Autodesk Inventor part; units mm, degrees
ref_plane "YZ Plane" through (0, 0, 0) normal (1, 0, 0) x (0, 1, 0)
ref_plane "XZ Plane" through (0, 0, 0) normal (0, 1, 0) x (-1, 0, 0)
ref_plane "XY Plane" through (0, 0, 0) normal (0, 0, 1) x (1, 0, 0)
sketch "Sketch1" plane through (0, 0, 0) normal (0, 1, 0) x (-1, 0, 0)
  circle A0 centre (0, 0) radius 1.1
  dimension "d0" = 2.2
extrude "Extrusion1" add sketch "Sketch1" along normal blind 16
sketch "Sketch2" plane through (0, 16, 0) normal (0, 1, 0) x (1, 0, 0)
  circle A0 centre (0, 0) radius 1.85
  dimension "d3" = 3.7
extrude "Extrusion2" add sketch "Sketch2" along normal blind 1.5
fillet "Fillet1" radius 0.5 1 edges at (-1.85, 17.5, 0)
sketch "Sketch3" plane through (0, 17.5, 0) normal (0, 1, 0) x (1, 0, 0)
  line L0 (0.3, -0.9) -> (-0.3, -0.9)
  line L1 (-0.3, 0.9) -> (0.3, 0.9)
  line L2 (0.3, -0.9) -> (-0.3, 0.9) construction
  line L3 (-0.3, -0.9) -> (0.3, 0.9) construction
  line L4 (-0.9, 0.3) -> (-0.9, -0.3)
  line L5 (0.9, -0.3) -> (0.9, 0.3)
  line L6 (0.9, 0.3) -> (-0.9, -0.3) construction
  line L7 (-0.9, 0.3) -> (0.9, -0.3) construction
  line L8 (-0.3, -0.9) -> (-0.3, -0.3)
  line L9 (-0.3, 0.3) -> (-0.3, 0.9)
  line L10 (0.3, 0.9) -> (0.3, 0.3)
  line L11 (0.3, -0.3) -> (0.3, -0.9)
  line L12 (-0.9, -0.3) -> (-0.3, -0.3)
  line L13 (0.3, -0.3) -> (0.9, -0.3)
  line L14 (-0.3, 0.3) -> (-0.9, 0.3)
  line L15 (0.9, 0.3) -> (0.3, 0.3)
  point P0 (0, 0)
  dimension "d7" = 0.6
  dimension "d8" = 1.8
  dimension "d9" = 1.8
  dimension "d10" = 0.6
  dimension "d11" = 0.6
  dimension "d12" = 0.6
  dimension "d13" = 0.6
  dimension "d14" = 0.6
extrude "Extrusion3" cut sketch "Sketch3" against normal blind 1.5
chamfer "Chamfer1" distance 0.5 angle 45 1 edges at (1.1, 0, 0)
properties part number "screwKa22x16"
Design review of the part built by this model. Coordinates are the model's own, in mm. A direction names the side the tool comes from. Give positions to 0.01 mm unless a question says otherwise; leave off trailing zeros. Order: outer loops, then holes, each group sorted by start corner. A loop starts at its lowest first (then second) coordinate and runs counter-clockwise, first axis right, second up. Notation, with made-up numbers: M 16,-8 L 23,-8 A24 cw 23,25 Z; hole C -33,29.25 d4. An arc over 180 degrees is marked long. One line per question, with ' | ' between items. Start each with the question number.
Q1. For pin 1 Ø1.4 at (x, z) = (-0.5, 0) entering from +Y; pin 2 Ø0.5 at (x, y) = (0.5, 16.5) entering from +Z; pin 3 Ø0.5 at (x, y) = (-0.5, 17) entering from -Z; pin 4 Ø1.5 at (x, y) = (0.5, 15) entering from -Z, all flat-tipped, find the tip position at first contact; note any pin that passes through.
Q2. We need section B-B (z = 0). Write out the cut boundary in (x, y), plus the area to 3 significant figures.
Q3. For L1, parallel to Y at x = 0, z = 0.2; L2, parallel to Z at x = 0.05, y = 3.75; L3, parallel to X at y = 16.75, z = -0.4, list the stretches that pass through material, from the lowest coordinate up. Write a range as [from, to].
Q4. We need section A-A (y = 16.5). Write out the cut boundary in (x, z).
Q5. Machinability: for faces 4 (the face through (1, 16, 1)), 5 (the face through (-0.6, 17.5, -0.6)), which of the approach directions +Z, -Z, +X, -X, +Y, -Y give a long, thin tool a straight path to every point of the face, cutting with its end or side? Answer none if there is none.
Q6. We need section D-D (y = 14.75). Write out the cut boundary in (x, z).
Q7. The part is to be moulded in two halves that separate along X. For faces 1 (the face through (0, 0, 0)), 2 (the face through (-1.05, 8.14, -0.33)), 3 (the face through (0, 16, 0)), say which applies: +X half, -X half, draft (parallel to the pull), parting line (faces both ways), or undercut.
Q8. We need section C-C (x = 0). Write out the cut boundary in (y, z).
Returned:
1) pin 1: y = 17.5 | pin 2: z = 1.83 | pin 3: z = -1.83 | pin 4: z = -1.1
2) outline: M -1.85,16 L -1.1,16 L -1.1,0.5 L -0.6,0 L 0.6,0 L 1.1,0.5 L 1.1,16 L 1.85,16 L 1.85,17 A0.5 ccw 1.35,17.5 L 0.9,17.5 L 0.9,16 L -0.9,16 L -0.9,17.5 L -1.35,17.5 A0.5 ccw -1.85,17 Z | area: 37.7 mm2
3) L1: [0, 16] | L2: [-1.1, 1.1] | L3: [-1.81, -0.3], [0.3, 1.81]
4) outline: C 0,0 d3.7; hole M -0.9,-0.3 L -0.3,-0.3 L -0.3,-0.9 L 0.3,-0.9 L 0.3,-0.3 L 0.9,-0.3 L 0.9,0.3 L 0.3,0.3 L 0.3,0.9 L -0.3,0.9 L -0.3,0.3 L -0.9,0.3 Z
5) face 4: -Y | face 5: +Z, -Z, +X, -X, +Y
6) outline: C 0,0 d2.2
7) face 1: draft | face 2: parting line | face 3: undercut
8) outline: M 0,-0.6 L 0.5,-1.1 L 16,-1.1 L 16,-1.85 L 17,-1.85 A0.5 ccw 17.5,-1.35 L 17.5,-0.9 L 16,-0.9 L 16,0.9 L 17.5,0.9 L 17.5,1.35 A0.5 ccw 17,1.85 L 16,1.85 L 16,1.1 L 0.5,1.1 L 0,0.6 Z
